from build123d import *

# Parameters (mm, degrees)
F0_R     = 1.778
F1_DEPTH = 3.175
F0_W     = 3.175
F0_H     = 12.7
F2_DEPTH = 25.4


with BuildPart() as f1:
    # F0 (on Right) → F1 (new body)
    with BuildSketch(Plane.YZ):
        Polygon((-63.5, 0), (0, 0), (0, 12.7), (-3.175, 12.7), (-3.175, 25.4), (0, 25.4), (0, 38.1), (-63.5, 38.1), align=None)
        with Locations((-22.5806, 9.525)):
            Circle(F0_R, mode=Mode.SUBTRACT)
        Polygon((-127, 0), (-63.5, 0), (-63.5, 38.1), (-127, 38.1), (-127, 25.4), (-123.825, 25.4), (-123.825, 12.7), (-127, 12.7), align=None)
        with Locations((-104.4194, 9.525)):
            Circle(F0_R, mode=Mode.SUBTRACT)
    extrude(amount=F1_DEPTH)

    # F0 (on Right) → F2 (cut)
    with BuildSketch(Plane.YZ):
        with Locations((-1.5875, 19.05)):
            Rectangle(F0_W, F0_H)
        with Locations((-125.4125, 19.05)):
            Rectangle(F0_W, F0_H)
    extrude(amount=-F2_DEPTH, mode=Mode.SUBTRACT)


solid = f1.part
The model under review builds one solid part; all positions refer to its coordinate system, in mm. A direction names the side the tool comes from. Round coordinates to 2 decimals unless told otherwise and drop trailing zeros. Loops run counter-clockwise (first coordinate to the right, second up) from the corner with the lowest first, then second, coordinate; pieces in that order, holes last. Notation, with made-up numbers: (24.5, 76.25) -> (34.5, 76.25) arc R22 ccw to (34.5, 111.25) -> close; hole circle Ø4 at (14.5, -2). An arc over 180 degrees is marked (long way). Write item = value, one per line. Start each with the question number.
Item 1: Take a section at C-C on z = 22. Give the boundary of the cut face in (x, y) (3 decimals).
Item 2: Take a section at B-B on x = 1.75. Give the boundary of the cut face in (y, z) (3 decimals).
Item 3: Mouldability with a two-part tool opening along Z and no side actions: class faces 4 (the cylindrical face through (1.565, -24.357, 9.603)), 5 (the flat face through (2, 0, 32)), 6 (the cylindrical face through (1.565, -102.724, 10.059)), 7 (the flat face through (2, -64, 0)) as released by +Z, released by -Z, zero draft, split by the parting line, or undercut.
Item 4: For faces 1 (the flat face through (2, -2, 12.7)), 2 (the flat face through (2, -123.825, 19)), 3 (the flat face through (0, -64, 19)), list the 3-axis set-ups (+Z, -Z, +X, -X, +Y, -Y) from which the entire face can be reached by the end or side of a thin tool; tool diameter is ignored.
Item 5: Insertion check: pin 1 (4 mm diameter, centred on y = -104.42, z = 9.52, fed in from +X) (3 decimals); pin 2 (3 mm diameter, centred on y = -22.58, z = 9.52, fed in from -X); pin 3 (1 mm diameter, centred on x = 1, z = 22, fed in from +Y) (3 decimals). Each pin has a flat end and moves straight along its axis. Give the tip position at first contact, or say it passes through.
Item 6: Take a section at A-A on y = -22.5. Give the boundary of the cut face in (x, z) (3 decimals), plus the area to 3 significant figures.
Item 7: To check wall thickness, follow L1, parallel to Y at x = 2.45, z = 16.5 (3 decimals); L2, parallel to Z at x = 2.05, y = -103. State the ranges of each line that lie inside material, in increasing order.
Result:
q1.outline = (0, -123.825) -> (3.175, -123.825) -> (3.175, -3.175) -> (0, -3.175) -> close
q2.outline = (-127, 0) -> (0, 0) -> (0, 12.7) -> (-3.175, 12.7) -> (-3.175, 25.4) -> (0, 25.4) -> (0, 38.1) -> (-127, 38.1) -> (-127, 25.4) -> (-123.825, 25.4) -> (-123.825, 12.7) -> (-127, 12.7) -> close; hole circle Ø3.556 at (-104.419, 9.525); hole circle Ø3.556 at (-22.581, 9.525)
q3.face_4 = undercut
q3.face_5 = zero draft
q3.face_6 = undercut
q3.face_7 = released by -Z
q4.face_1 = +X, -X, +Y
q4.face_2 = +X, -X, -Y
q4.face_3 = +Z, -Z, -X, +Y, -Y
q5.pin_1 = 3.175
q5.pin_2 = through
q5.pin_3 = -3.175
q6.outline = (0, 0) -> (3.175, 0) -> (3.175, 7.749) -> (0, 7.749) -> close; (0, 11.301) -> (3.175, 11.301) -> (3.175, 38.1) -> (0, 38.1) -> close
q6.area = 110 mm²
q7.L1 = -123.825 to -3.175
q7.L2 = 0 to 8.45, 10.6 to 38.1
